Input: part model. Units: mm. Frame: model coordinates. Face numbers are marked on the shaded views. A direction names the side the tool comes from. Give positions to 0.01 mm unless a question says otherwise; leave off trailing zeros. Write each loop counter-clockwise with the first axis right and the second up, starting at its lowest first coordinate (ties: lowest second). Pieces come first, ordered by that corner, then holes. Notation, with made-up numbers: (-8.75, 2.5) -> (23.25, 2.5) arc R22 ccw to (23.25, 18.5) -> close; hole circle Ø11 at (-13, 16). An arc over 180 degrees is marked (long way). Return JSON: item names as keys, results as strings. Group by question number.
Item 1: Section A-A, the plane z = -1.75. Return loops of the section in (x, y), then the cut area to 3 significant figures.
Item 2: Section D-D, the plane y = 19. Return loops of the section in (x, z).
Item 3: Section C-C, the plane z = 0. Return loops of the section in (x, y), then the cut area to 3 significant figures.
Item 4: Line query: line 1 (Y direction, x = -0.65, z = 1.1); line 2 (X direction, y = 2.5, z = 1); line 3 (X direction, y = 4, z = 2.3). Output: solid intervals per line, ascending. Write a range as [from, to].
Item 5: Set-up query: the marked faces 1, 2 and 3. Return all of +Z, -Z, +X, -X, +Y, -Y with unobstructed straight access to the full face (end or side cutting, diameter ignored); none if empty.
Item 6: Mould query, pull axis Z, two halves, no side actions, for the marked faces 4, 5, 6 and 7. Classes: released by +Z, released by -Z, zero draft, split by the parting line, or undercut.
Item 7: Section B-B, the plane x = -1.6. Return loops of the section in (y, z), then the cut area to 3 significant figures.
Item 8: Pin query (flat end, axial travel): P1, Ø1.5, axis at x = 1.5, y = 5, coming from the -Z side. Return the tip coordinate at first contact, or that it passes through.
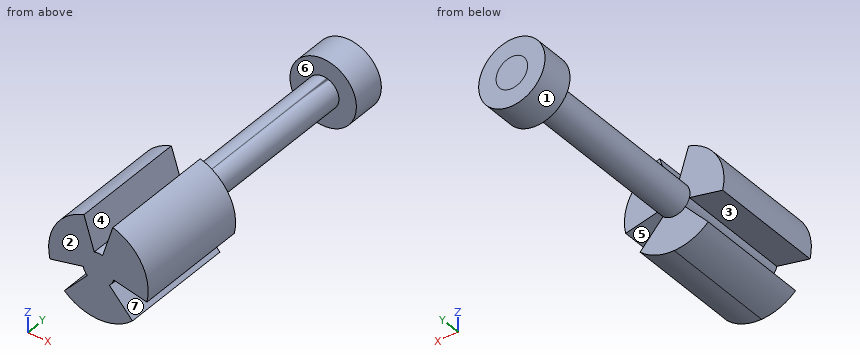
from build123d import *
from build123d.topology import SkipClean

# Parameters (mm, degrees)
SKETCH1_R           = 0.95
BOSS_EXTRUDE1_DEPTH = 20
SKETCH2_R           = 3
SKETCH2_R_2         = 0.95
BOSS_EXTRUDE2_DEPTH = 7
CUT_EXTRUDE1_DEPTH  = 14.674794331
CIRPATTERN1_COUNT   = 3
SKETCH5_R           = 2
BOSS_EXTRUDE3_DEPTH = 2


with BuildPart() as part:
    # Sketch1 → Boss-Extrude1 (new body)
    with BuildSketch(Plane(origin=(0, 0, 0), x_dir=(1, 0, 0), z_dir=(0, 1, 0))):
        with Locations(Location((0, 0, 0), (0, 0, 270))):
            Circle(SKETCH1_R)
    extrude(amount=BOSS_EXTRUDE1_DEPTH)

    # Sketch2 → Boss-Extrude2 (add)
    with BuildSketch(Plane.XZ):
        with Locations(Location((0, 0, 0), (0, 0, 270))):
            Circle(SKETCH2_R)
        with Locations(Location((0, 0, 0), (0, 0, 270))):
            Circle(SKETCH2_R_2, mode=Mode.SUBTRACT)
    extrude(amount=-BOSS_EXTRUDE2_DEPTH)

    # Sketch3 → Cut-Extrude1 (cut, through all)
    with SkipClean():  # the faces are left unmerged after this step: merging them gives an invalid solid
        with BuildSketch(Plane(origin=(0, 7, 0), x_dir=(1, 0, 0), z_dir=(0, 1, 0))):
            with BuildLine():
                Line((0.25, -0.916515139), (1.158545021, -3.775631426))
                Line((1.158545021, -3.775631426), (-1.158545021, -3.775631426))
                Line((-1.158545021, -3.775631426), (-0.25, -0.916515139))
                ThreePointArc((-0.25, -0.916515139), (0, -0.95), (0.25, -0.916515139))
            make_face()
        cut_extrude1 = extrude(amount=-CUT_EXTRUDE1_DEPTH, mode=Mode.SUBTRACT)

    # CirPattern1: Cut-Extrude1 ×3 about axis
    with SkipClean():  # the faces are left unmerged after this step: merging them gives an invalid solid
        cirpattern1_axis = Axis((0, 0, 0), (0, 1, 0))
        for i in range(1, CIRPATTERN1_COUNT):
            add(cut_extrude1.rotate(cirpattern1_axis, i * 360 / CIRPATTERN1_COUNT), mode=Mode.SUBTRACT)

    # Sketch5 → Boss-Extrude3 (add)
    with SkipClean():  # the faces are left unmerged after this step: merging them gives an invalid solid
        with BuildSketch(Plane(origin=(0, 18, 0), x_dir=(1, 0, 0), z_dir=(0, 1, 0))):
            with Locations(Location((0, 0, 0), (0, 0, 270))):
                Circle(SKETCH5_R)
        extrude(amount=BOSS_EXTRUDE3_DEPTH)


solid = part.part
Answer below:
{
 "1": {"outline": "(-1.65, 0) -> (1.65, 0) -> (1.65, 7) -> (-1.65, 7) -> close; (-0.97, 18) -> (0.97, 18) -> (0.97, 20) -> (-0.97, 20) -> close", "area": "27.0 mm2"},
 "2": {"outline": "circle Ø4 at (0, 0)"},
 "3": {"outline": "(-3, 0) -> (3, 0) -> (3, 7) -> (0.95, 7) -> (0.95, 18) -> (2, 18) -> (2, 20) -> (-2, 20) -> (-2, 18) -> (-0.95, 18) -> (-0.95, 7) -> (-3, 7) -> close", "area": "70.9 mm2"},
 "4": {"line 1": "y = [0, 7], [18, 20]", "line 2": "x = [-2.83, -0.28], [0.28, 2.83]", "line 3": "x = [-1.93, -0.69], [0.69, 1.93]"},
 "5": {"face 1": "+Y", "face 2": "+Z, -Z, +X, -X, -Y", "face 3": "-Y"},
 "6": {"face 4": "released by +Z", "face 5": "undercut", "face 6": "zero draft", "face 7": "undercut"},
 "7": {"outline": "(0, -2.54) -> (7, -2.54) -> (7, -1.7) -> (0, -1.7) -> close; (0, -0.39) -> (7, -0.39) -> (7, 2.54) -> (0, 2.54) -> close; (18, -1.2) -> (20, -1.2) -> (20, 1.2) -> (18, 1.2) -> close", "area": "31.2 mm2"},
 "8": {"P1": "stops at z = -2.9"}
}
